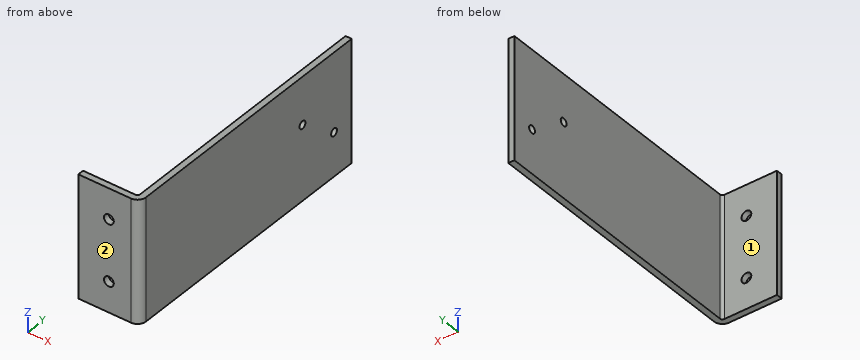
```python
from build123d import *

# Parameters (mm, degrees)
SKETCH2_W                    = 25.4
SKETCH2_H                    = 50.8
BASE_FLANGE1_DEPTH           = 2.54
EDGE_FLANGE1_STRIP_W         = 12.16
EDGE_FLANGE1_STRIP_H         = 2.54
EDGE_FLANGE1_STRIP_CUT_DEPTH = 50.8
EDGE_FLANGE1_DEPTH           = 50.8
SKETCH10_R                   = 2.032
CUT_EXTRUDE1_DEPTH           = 128.633420388
SKETCH11_R                   = 1.5748
CUT_EXTRUDE2_DEPTH           = 125.874005301


# Sheet-metal steps are written as plain solids
with BuildPart() as part:
    # Sketch2 → Base-Flange1 (new body)
    with BuildSketch(Plane(origin=(0, 0, 0), x_dir=(1, 0, 0), z_dir=(0, 1, 0))):
        with Locations((12.7, 25.4)):
            Rectangle(SKETCH2_W, SKETCH2_H)
    extrude(amount=-BASE_FLANGE1_DEPTH)

    # Edge-Flange1 strip (across the edge) → Edge-Flange1 strip cut (cut)
    with BuildSketch(Plane(origin=(25.4, 0, 0), x_dir=(-1, 0, 0), z_dir=(0, 0, -1))):
        with Locations((-2.54, -1.27)):
            Rectangle(EDGE_FLANGE1_STRIP_W, EDGE_FLANGE1_STRIP_H)
    extrude(amount=EDGE_FLANGE1_STRIP_CUT_DEPTH, mode=Mode.SUBTRACT)

    # Edge-Flange1 section (across the edge) → Edge-Flange1 (add)
    with BuildSketch(Plane(origin=(25.4, 0, 0), x_dir=(-1, 0, 0), z_dir=(0, 0, -1))):
        with BuildLine():
            Line((0, 1), (0, 111.76))
            Line((0, 111.76), (2.54, 111.76))
            Line((2.54, 111.76), (2.54, 1))
            ThreePointArc((2.54, 1), (2.832893219, 0.292893219), (3.54, 0))
            Line((3.54, 0), (3.54, -2.54))
            ThreePointArc((3.54, -2.54), (1.036841995, -1.503158005), (0, 1))
        make_face()
    extrude(amount=EDGE_FLANGE1_DEPTH)

    # Sketch10 → Cut-Extrude1 (cut, through all)
    with BuildSketch(Plane.XZ.offset(2.54)):
        with Locations(Location((12.7, -38.1, 0), (0, 0, 270))):
            Circle(SKETCH10_R)
        with Locations(Location((12.7, -12.7, 0), (0, 0, 270))):
            Circle(SKETCH10_R)
    extrude(amount=-CUT_EXTRUDE1_DEPTH, mode=Mode.SUBTRACT)

    # Sketch11 → Cut-Extrude2 (cut, through all)
    with BuildSketch(Plane.ZY.offset(-22.86)):
        with Locations(Location((-32.639, 102.2604, 0), (0, 0, 270))):
            Circle(SKETCH11_R)
        with Locations(Location((-19.685, 85.2424, 0), (0, 0, 270))):
            Circle(SKETCH11_R)
    extrude(amount=-CUT_EXTRUDE2_DEPTH, mode=Mode.SUBTRACT)


solid = part.part
```
The listing builds one solid part. Answer for the finished solid, in the listing's coordinates (mm). Face numbers are marked on the shaded views. A direction names the side the tool comes from. Give positions to 0.01 mm unless a question says otherwise; leave off trailing zeros. Order: outer loops, then holes, each group sorted by start corner. A loop starts at its lowest first (then second) coordinate and runs counter-clockwise, first axis right, second up. Notation, with made-up numbers: (-19, 25) -> (37, 25) arc R19 cw to (37, 32) -> close; hole circle Ø6 at (-24.75, 7). An arc over 180 degrees is marked (long way). Answer as CSV lines item,"result". Start each with the question number.
Q1. Find the intervals of material crossed by L1, parallel to X at y = 16.5, z = -37; L2, parallel to Y at x = 15.5, z = -29; L3, parallel to X at y = -1, z = -38.1, in increasing order.
Q2. A cutting plane is placed at A-A (x = 12.7). Determine the outline of the cut face in (y, z), then the cut area to 3 significant figures.
Q3. A cutting plane is placed at B-B (z = -38.1). Determine the outline of the cut face in (x, y), then the cut area to 3 significant figures.
Q4. A cutting plane is placed at C-C (z = -16). Determine the outline of the cut face in (x, y).
Q5. Given pin 1 (3 mm diameter, centred on y = 69, z = -25, fed in from -X); pin 2 (1.5 mm diameter, centred on x = 3.5, z = -26, fed in from +Y), each flat-ended and moving along its own axis, determine where each tip first touches the part or whether it passes through.
Q6. A cutting plane is placed at D-D (y = 9.5). Determine the outline of the cut face in (x, z).
Q7. Which of the six approach directions +Z, -Z, +X, -X, +Y, -Y give full straight-line access (tool end or side, diameter ignored) to the marked faces 1 and 2?
Results found:
1,L1,"22.86 to 25.4"
1,L2,"-2.54 to 0"
1,L3,"0 to 10.67, 14.73 to 24.78"
2,outline,"(-2.54, -50.8) -> (0, -50.8) -> (0, -40.13) -> (-2.54, -40.13) -> close; (-2.54, -36.07) -> (0, -36.07) -> (0, -14.73) -> (-2.54, -14.73) -> close; (-2.54, -10.67) -> (0, -10.67) -> (0, 0) -> (-2.54, 0) -> close"
2,area,"108 mm2"
3,outline,"(0, -2.54) -> (10.67, -2.54) -> (10.67, 0) -> (0, 0) -> close; (14.73, -2.54) -> (21.86, -2.54) arc R3.54 ccw to (25.4, 1) -> (25.4, 111.76) -> (22.86, 111.76) -> (22.86, 1) arc R1 cw to (21.86, 0) -> (14.73, 0) -> close"
3,area,"336 mm2"
4,outline,"(0, -2.54) -> (21.86, -2.54) arc R3.54 ccw to (25.4, 1) -> (25.4, 111.76) -> (22.86, 111.76) -> (22.86, 1) arc R1 cw to (21.86, 0) -> (0, 0) -> close"
5,pin 1,"x = 22.86"
5,pin 2,"y = 0"
6,outline,"(22.86, -50.8) -> (25.4, -50.8) -> (25.4, 0) -> (22.86, 0) -> close"
7,face 1,"+Z, -Z, -X, +Y"
7,face 2,"+Z, -Z, +X, -X, -Y"
